```python
from build123d import *


with BuildPart() as part:
    # Sketch1 → Revolve1 (revolve)
    with BuildSketch(Plane.XY):
        with BuildLine():
            Line((-16.933310091, 12.7), (-10.68830568, 8.01622926))
            ThreePointArc((-10.68830568, 8.01622926), (-7.738067215, 4.481206386), (-6.6802, 0))
            Line((-6.6802, 0), (-6.6802, -3.175))
            Line((-6.6802, -3.175), (-8.621589827, -9.525))
            Line((-8.621589827, -9.525), (-15.24, -9.525))
            Line((-15.24, -9.525), (-21.59, -3.175))
            Line((-21.59, -3.175), (-21.59, 12.7))
            Line((-21.59, 12.7), (-16.933310091, 12.7))
        make_face()
    revolve(axis=Axis((0, 0, 0), (0, 1, 0)))


solid = part.part
```
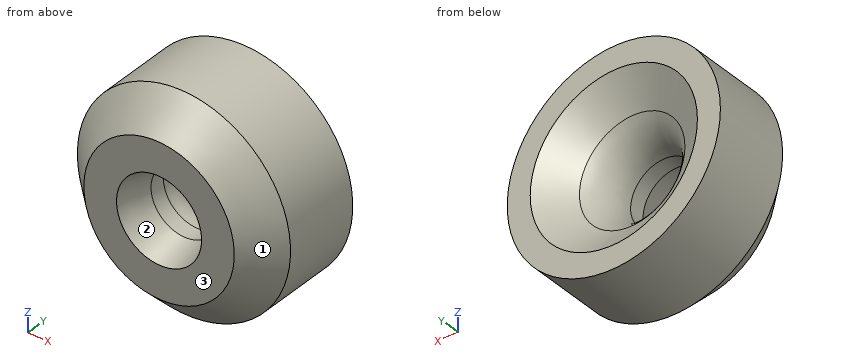
Check sheet for the modelled part. Datum: model origin and axes. Units: mm. Face numbers are marked on the shaded views. Round coordinates to 2 decimals unless told otherwise and drop trailing zeros. Order: outer loops, then holes, each group sorted by start corner. A loop starts at its lowest first (then second) coordinate and runs counter-clockwise, first axis right, second up.
1) Go/stop test with flat-tipped pins: pin 1 Ø2 at (x, y) = (16, 8) entering from -Z; pin 2 Ø4 at (y, z) = (6, -9) entering from +X; pin 3 Ø4 at (x, y) = (-9, -5.5) entering from -Z. Record where each tip stops, or that it passes through.
2) Section check D-D (y = -5.75). Record the boundary of the cut face in (x, z) (3 decimals).
3) Scan lines: line 1 (Z direction, x = 0, y = -1.7); line 2 (Z direction, x = 0, y = -4.5) (3 decimals); line 3 (X direction, y = 5.5, z = 1.5). Record each from-to range of solid material in increasing order.
4) Mould release check, pull along X, two halves, no side actions. Record for the marked faces 1, 2 and 3: +X half, -X half, draft (parallel to the pull), parting line (faces both ways), or undercut.
5) Section check C-C (y = -2.25). Record the boundary of the cut face in (x, z).
6) Section check B-B (z = 0). Record the boundary of the cut face in (x, y) (1 decimal).
7) Section check A-A (x = 0). Record the boundary of the cut face in (y, z) (1 decimal), and give its area (3 significant figures).
Result:
1. pin 1: stops at z = -15.53
1. pin 2: stops at x = 20.42
1. pin 3: stops at z = -19.44
2. outline: circle Ø38.03 at (0, 0); hole circle Ø14.935 at (0, 0)
3. line 1: z = -21.59 to -6.68, 6.68 to 21.59
3. line 2: z = -20.265 to -7.085, 7.085 to 20.265
3. line 3: x = -21.54 to -8.19, 8.19 to 21.54
4. face 1: parting line
4. face 2: undercut
4. face 3: draft
5. outline: circle Ø43.18 at (0, 0); hole circle Ø13.36 at (0, 0)
6. outline: (-21.6, -3.2) - (-15.2, -9.5) - (-8.6, -9.5) - (-6.7, -3.2) - (-6.7, 0) arc R10 ccw to (-10.7, 8) - (-16.9, 12.7) - (-21.6, 12.7) - close; (6.7, -3.2) - (8.6, -9.5) - (15.2, -9.5) - (21.6, -3.2) - (21.6, 12.7) - (16.9, 12.7) - (10.7, 8) arc R10 ccw to (6.7, 0) - close
7. outline: (-9.5, -15.2) - (-3.2, -21.6) - (12.7, -21.6) - (12.7, -16.9) - (8, -10.7) arc R10 ccw to (0, -6.7) - (-3.2, -6.7) - (-9.5, -8.6) - close; (-9.5, 8.6) - (-3.2, 6.7) - (0, 6.7) arc R10 ccw to (8, 10.7) - (12.7, 16.9) - (12.7, 21.6) - (-3.2, 21.6) - (-9.5, 15.2) - close
7. area: 524 mm2
